from build123d import *

# Parameters (mm, degrees)
F0_W     = 58.5
F0_H     = 73.5
F0_R     = 2.5
F1_DEPTH = 20
F2_W     = 47
F2_H     = 12
F2_W_2   = 4
F3_DEPTH = 6.5


with BuildPart() as f1:
    # F0 (on Top) → F1 (new body)
    with BuildSketch(Plane.XY):
        with Locations((9.048133, -1.976883)):
            Rectangle(F0_W, F0_H)
        with Locations((3.298133, -27.226883)):
            Circle(F0_R, mode=Mode.SUBTRACT)
        Polygon((14.798133, 21.773117), (21.798133, 21.773117), (31.798133, 21.773117), (31.798133, -33.226883), (21.798133, -33.226883), (21.798133, -19.226883), (14.798133, -19.226883), (14.798133, -27.226883), (11.798133, -27.226883), (11.798133, -19.226883), (3.298133, -19.226883), (-1.701867, -19.226883), (-8.201867, -26.226883), (-15.201867, -26.226883), (-15.201867, -19.226883), (-15.201867, 21.773117), (3.298133, 21.773117), (11.798133, 21.773117), (11.798133, 29.773117), (14.798133, 29.773117), align=None, mode=Mode.SUBTRACT)
        with Locations((3.298133, 27.773117)):
            Circle(F0_R, mode=Mode.SUBTRACT)
    extrude(amount=F1_DEPTH)

    # F2 (on face) → F3 (cut, through all)
    with BuildSketch(Plane.YZ.offset(38.298133)):
        with Locations((-5.726883, 6)):
            Rectangle(F2_W, F2_H)
        with Locations((19.773117, 6)):
            Rectangle(F2_W_2, F2_H)
    extrude(amount=-F3_DEPTH, mode=Mode.SUBTRACT)


solid = f1.part
Build history of the part. All positions in model axes, mm. A direction names the side the tool comes from. Round coordinates to 2 decimals unless told otherwise and drop trailing zeros. Write each loop counter-clockwise with the first axis right and the second up, starting at its lowest first coordinate (ties: lowest second). Pieces come first, ordered by that corner, then holes. Notation, with made-up numbers: (-6, 1) - (1, 1) arc R30 ccw to (1, 37) - close; hole circle Ø8 at (48.5, 28.5). An arc over 180 degrees is marked (long way). One line per question, with ' | ' between items.
1. Band-saw the part on D-D, the plane x = 3. Write the cut outline in (y, z), and give its area (3 significant figures).
Results are:
outline: (-38.73, 0) - (-29.71, 0) - (-29.71, 20) - (-38.73, 20) - close; (-24.74, 0) - (-19.23, 0) - (-19.23, 20) - (-24.74, 20) - close; (21.77, 0) - (25.29, 0) - (25.29, 20) - (21.77, 20) - close; (30.26, 0) - (34.77, 0) - (34.77, 20) - (30.26, 20) - close | area: 451 mm^2
2. Tool access for faces 4 (the face through (35, -29.227, 6)), 5 (the face through (13, 29.773, 10)), 6 (the face through (9, 34.773, 10)): list every direction of +Z, -Z, +X, -X, +Y, -Y with a clear straight run to the whole face (end or side of a thin tool).
Results are:
face 4: -Z, +X | face 5: +Z, -Z | face 6: +Z, -Z, +X, -X, +Y
3. Mould opens along X. For faces 1 (the face through (14.798, 26, 10)), 2 (the face through (35, -3, 12)), 3 (the face through (-20.202, -2, 10)) say: released by +X, released by -X, zero draft, split by the parting line, or undercut.
Results are:
face 1: undercut | face 2: zero draft | face 3: released by -X
4. Band-saw the part on C-C, the plane z = 9.75. Write the cut outline in (x, y), and give its area (3 significant figures).
Results are:
outline: (-20.2, -38.73) - (38.3, -38.73) - (38.3, -29.23) - (31.8, -29.23) - (31.8, -33.23) - (21.8, -33.23) - (21.8, -19.23) - (14.8, -19.23) - (14.8, -27.23) - (11.8, -27.23) - (11.8, -19.23) - (-1.7, -19.23) - (-8.2, -26.23) - (-15.2, -26.23) - (-15.2, 21.77) - (11.8, 21.77) - (11.8, 29.77) - (14.8, 29.77) - (14.8, 21.77) - (38.3, 21.77) - (38.3, 34.77) - (-20.2, 34.77) - close; hole circle Ø5 at (3.3, -27.23); hole circle Ø5 at (3.3, 27.77) | area: 1,740 mm^2
5. Drill centre lines: line 1 along Y through (x, z) = (-9.5, 18.75); line 2 along X through (y, z) = (9.5, 14); line 3 along Y through (x, z) = (22, 2). Where is each one in solid material? Low to high. Write a range as from..to.
Results are:
line 1: -38.73..-26.23, 21.77..34.77 | line 2: -20.2..-15.2, 31.8..38.3 | line 3: -38.73..-33.23, 21.77..34.77
6. Band-saw the part on B-B, the plane x = 11. Write the cut outline in (y, z).
Results are:
outline: (-38.73, 0) - (-19.23, 0) - (-19.23, 20) - (-38.73, 20) - close; (21.77, 0) - (34.77, 0) - (34.77, 20) - (21.77, 20) - close
7. Drop flat-ended pins along their axis: pin 1 Ø6 at (x, y) = (3.3, -27.23) entering from +Z; pin 2 Ø7 at (x, y) = (34, -10.5) entering from -Z; pin 3 Ø6.5 at (y, z) = (-22.5, 5.5) entering from +X. Give the stop position or say it passes through.
Results are:
pin 1: z = 20 | pin 2: z = 12 | pin 3: x = 21.8
8. Band-saw the part on A-A, the plane y = 0.5. Write the cut outline in (x, z).
Results are:
outline: (-20.2, 0) - (-15.2, 0) - (-15.2, 20) - (-20.2, 20) - close; (31.8, 12) - (38.3, 12) - (38.3, 20) - (31.8, 20) - close
